Part model, mm, in its own coordinate system. Face numbers are marked on the shaded views. A direction names the side the tool comes from. Give positions to 0.01 mm unless a question says otherwise; leave off trailing zeros. Write each loop counter-clockwise with the first axis right and the second up, starting at its lowest first coordinate (ties: lowest second). Pieces come first, ordered by that corner, then holes. Notation, with made-up numbers: M 66,73 L 79,73 A30 cw 79,107 Z; hole C 88.5,72.25 d5. An arc over 180 degrees is marked long. Use CSV: the item, a comma, the result in double quotes. Start each with the question number.
1. Drill centre lines: line 1 along X through (y, z) = (21, 12.25); line 2 along Y through (x, z) = (-10, 18.9); line 3 along Y through (x, z) = (-16, 1.75). Where is each one in solid material? Low to high. Write a range as from..to.
2. Band-saw the part on C-C, the plane z = 3.5. List the corners of the cut face in (x, y), then the cut area to 3 significant figures.
3. Band-saw the part on D-D, the plane y = 29. List the corners of the cut face in (x, z), then the cut area to 3 significant figures.
4. Band-saw the part on B-B, the plane y = 16.5. List the corners of the cut face in (x, z).
5. 3-axis set-ups, long thin cutter, end or side, ignore diameter. For the marked faces 5 and 6: which of +Z, -Z, +X, -X, +Y, -Y reach the whole face in a straight line?
6. Mould opens along X. For the marked faces 1, 2, 3 and 4 say: pulls with the +X half, pulls with the -X half, needs draft (parallel to the pull), parting line crosses it, or undercut.
7. Band-saw the part on A-A, the plane x = -10. List the corners of the cut face in (y, z), then the cut area to 3 significant figures.
8. Drop flat-ended pins along their axis: pin 1 Ø1.6 at (x, y) = (-9, 32) entering from -Z; pin 2 Ø8 at (x, y) = (-8.5, 21) entering from -Z; pin 3 Ø5.5 at (x, y) = (-10, 16.5) entering from -Z. Give the stop position or say it passes through.
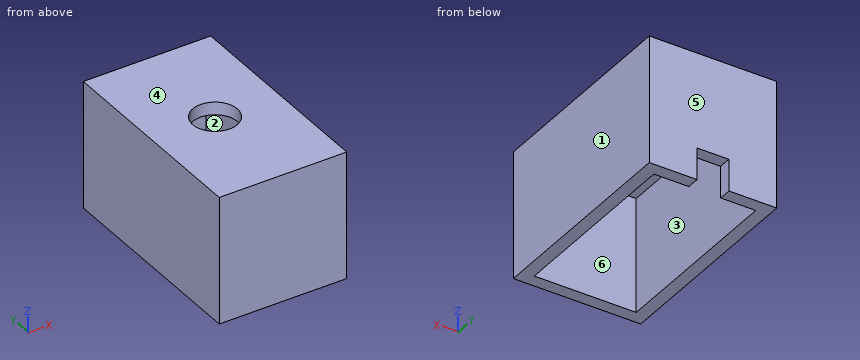
from build123d import *

# Parameters (mm, degrees)
F0_W     = 20
F0_H     = 33
F0_R     = 3.5
F1_DEPTH = 20
F2_W     = 16
F2_H     = 29
F2_R     = 3.5
F3_DEPTH = 18
F4_W     = 5
F4_H     = 2
F5_DEPTH = 5


with BuildPart() as f1:
    # F0 (on Top) → F1 (new body)
    with BuildSketch(Plane.XY):
        with Locations((-10, 16.5)):
            Rectangle(F0_W, F0_H)
        with Locations((-10, 16.5)):
            Circle(F0_R, mode=Mode.SUBTRACT)
    extrude(amount=F1_DEPTH)

    # F2 (on face) → F3 (cut)
    with BuildSketch(Plane(origin=(0, 0, 0), x_dir=(1, 0, 0), z_dir=(0, 0, -1))):
        with Locations((-10, -16.5)):
            Rectangle(F2_W, F2_H)
        with Locations((-10, -16.5)):
            Circle(F2_R, mode=Mode.SUBTRACT)
    extrude(amount=-F3_DEPTH, mode=Mode.SUBTRACT)

    # F4 (on face) → F5 (cut)
    with BuildSketch(Plane(origin=(0, 0, 0), x_dir=(1, 0, 0), z_dir=(0, 0, -1))):
        with Locations((-10, -32)):
            Rectangle(F4_W, F4_H)
    extrude(amount=-F5_DEPTH, mode=Mode.SUBTRACT)


solid = f1.part
Output:
1,line 1,"x = -20..-18, -2..0"
1,line 2,"y = 0..13, 20..33"
1,line 3,"y = 0..2, 31..33"
2,outline,"M -20,0 L 0,0 L 0,33 L -7.5,33 L -7.5,31 L -2,31 L -2,2 L -18,2 L -18,31 L -12.5,31 L -12.5,33 L -20,33 Z"
2,area,"186 mm²"
3,outline,"M -20,0 L -18,0 L -18,18 L -2,18 L -2,0 L 0,0 L 0,20 L -20,20 Z"
3,area,"112 mm²"
4,outline,"M -20,0 L -18,0 L -18,18 L -13.5,18 L -13.5,20 L -20,20 Z; M -6.5,18 L -2,18 L -2,0 L 0,0 L 0,20 L -6.5,20 Z"
5,face 5,"+Z, -Z, +X, -X, +Y"
5,face 6,"-Z"
6,face 1,"pulls with the +X half"
6,face 2,"undercut"
6,face 3,"undercut"
6,face 4,"needs draft"
7,outline,"M 0,0 L 2,0 L 2,18 L 13,18 L 13,20 L 0,20 Z; M 20,18 L 31,18 L 31,5 L 33,5 L 33,20 L 20,20 Z"
7,area,"114 mm²"
8,pin 1,"stops at z = 5"
8,pin 2,"stops at z = 18"
8,pin 3,"passes through"
